Verification items for the finished model (mm, model axes). Face numbers are marked on the shaded views. A direction names the side the tool comes from. Round coordinates to 2 decimals unless told otherwise and drop trailing zeros. Order: outer loops, then holes, each group sorted by start corner. A loop starts at its lowest first (then second) coordinate and runs counter-clockwise, first axis right, second up. Notation, with made-up numbers: (76, 4) -> (127, 4) arc R10 cw to (127, 21) -> close; hole circle Ø9 at (84, -39). An arc over 180 degrees is marked (long way). Put each result on its own line as item: value.
Autodesk Inventor part; units mm, degrees
ref_plane "YZ Plane" through (0, 0, 0) normal (1, 0, 0) x (0, 1, 0)
ref_plane "XZ Plane" through (0, 0, 0) normal (0, 1, 0) x (-1, 0, 0)
ref_plane "XY Plane" through (0, 0, 0) normal (0, 0, 1) x (1, 0, 0)
sketch "Sketch_1" plane through (0, 0, 0) normal (1, 0, 0) x (0, 1, 0)
  line L0 (0, 50.8) -> (0, 0)
  line L1 (0, 0) -> (25.4, 0)
  arc A0 (25.4, 0) -> (20.6502, 4.7498) centre (20.6502, 0) ccw
  line L2 (20.6502, 4.7498) -> (7.9248, 4.7498)
  arc A1 (4.7498, 7.9248) -> (7.9248, 4.7498) centre (7.9248, 7.9248) ccw
  line L3 (4.7498, 7.9248) -> (4.7498, 46.0502)
  arc A2 (4.7498, 46.0502) -> (0, 50.8) centre (0, 46.0502) ccw
extrude "Extrusion1" add sketch "Sketch_1" along normal mid plane 22.225
sketch "Sketch_2" plane through (0, 0, 0) normal (0, 0, 1) x (1, 0, 0)
  arc A0 (-3.5687, 12.7) -> (3.5687, 12.7) centre (0, 12.7) ccw
  line L0 (3.5687, 12.7) -> (3.5687, 17.4752)
  arc A1 (3.5687, 17.4752) -> (-3.5687, 17.4752) centre (0, 17.4752) ccw
  line L1 (-3.5687, 17.4752) -> (-3.5687, 12.7)
extrude "Extrusion2" cut sketch "Sketch_2" along normal blind 7.9248
sketch "Sketch3" plane through (-11.1125, 0, 50.8) normal (0, -1, 0) x (1, 0, 0)
  point P0 (11.1125, -38.1)
hole "Hole1" at (0, 0, 12.7) direction (0, 1, 0) diameter 7.1374 depth 7.9248
sketch "Sketch4" plane through (-11.1125, 0, 50.8) normal (0, -1, 0) x (1, 0, 0)
  point P0 (11.1125, -12.7)
hole "Hole2" at (0, 0, 38.1) direction (0, 1, 0) diameter 7.1374 depth 7.9248
properties part number "4250"
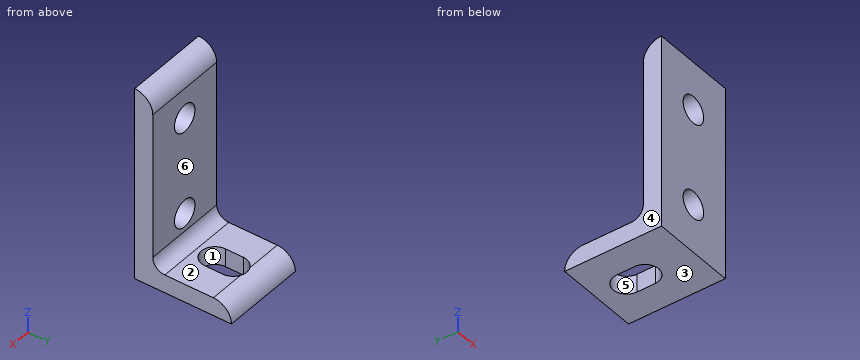
Item 1: Sectioned sample at A-A, the plane z = 38.1. Record the boundary of the cut face in (x, y), then the cut area to 3 significant figures.
Geometry check:
outline: (-11.11, 0) -> (-3.57, 0) -> (-3.57, 4.75) -> (-11.11, 4.75) -> close; (3.57, 0) -> (11.11, 0) -> (11.11, 4.75) -> (3.57, 4.75) -> close
area: 71.7 mm2
Item 2: Sectioned sample at C-C, the plane x = 7.75. Record the boundary of the cut face in (y, z) (3 decimals), then the cut area to 3 significant figures.
Geometry check:
outline: (0, 0) -> (25.4, 0) arc R4.75 ccw to (20.65, 4.75) -> (7.925, 4.75) arc R3.175 cw to (4.75, 7.925) -> (4.75, 46.05) arc R4.75 ccw to (0, 50.8) -> close
area: 332 mm2
Item 3: Material ranges on line 1 along X through (y, z) = (1.7, 38.1); line 2 along Z through (x, y) = (0, 3.05); line 3 along Z through (x, y) = (2.5, 2), recorded low to high.
Geometry check:
line 1: -11.11 to -3.57, 3.57 to 11.11
line 2: 0 to 9.13, 16.27 to 34.53, 41.67 to 49.69
line 3: 0 to 10.15, 15.25 to 35.55, 40.65 to 50.36
Item 4: Sectioned sample at D-D, the plane y = 20. Record the boundary of the cut face in (x, z).
Geometry check:
outline: (-11.11, 0) -> (-2.52, 0) -> (-2.52, 4.75) -> (-11.11, 4.75) -> close; (2.52, 0) -> (11.11, 0) -> (11.11, 4.75) -> (2.52, 4.75) -> close
Item 5: Release check for a two-part mould opening along Y. For the marked faces 4, 5 and 6 record: pulls with the +Y half, pulls with the -Y half, needs draft (parallel to the pull), parting line crosses it, or undercut.
Geometry check:
face 4: needs draft
face 5: undercut
face 6: pulls with the +Y half
Item 6: Sectioned sample at B-B, the plane x = 0. Record the boundary of the cut face in (y, z) (3 decimals).
Geometry check:
outline: (0, 0) -> (9.131, 0) -> (9.131, 4.75) -> (7.925, 4.75) arc R3.175 cw to (4.75, 7.925) -> (4.75, 9.131) -> (0, 9.131) -> close; (0, 16.269) -> (4.75, 16.269) -> (4.75, 34.531) -> (0, 34.531) -> close; (0, 41.669) -> (4.75, 41.669) -> (4.75, 46.05) arc R4.75 ccw to (0, 50.8) -> close; (21.044, 0) -> (25.4, 0) arc R4.75 ccw to (21.044, 4.733) -> close
Item 7: Depth check by flat-ended pin: pin 1 Ø6.5 at (x, y) = (-0.5, 12.5) entering from +Z; pin 2 Ø1 at (x, y) = (-2, 12.5) entering from +Z; pin 3 Ø11 at (x, z) = (0, 19) entering from +Y. Enter the tip coordinate at first touch or a pass-through.
Geometry check:
pin 1: z = 4.75
pin 2: through
pin 3: y = 4.75
Item 8: Tool access check on the marked faces 1, 2 and 3. Record the directions out of +Z, -Z, +X, -X, +Y, -Y that give a thin tool (end or side, any length) a straight path to the whole face; none if there is none.
Geometry check:
face 1: +Z, -Z
face 2: +Z, +X, -X, +Y
face 3: -Z, +X, -X, +Y, -Y
